Could you check a few things on this drawing? It's one solid part, dimensions in mm from its lowest x, y, z. A direction names the side the tool comes from. Coordinates: 2 decimals unless noted, no trailing zeros. Order: outer loops, then holes, each group sorted by start corner. A loop starts at its lowest first (then second) coordinate and runs counter-clockwise, first axis right, second up. Notation, with made-up numbers: (83, 6) - (101, 6) arc R21 ccw to (101, 30) - close; hole circle Ø2 at (-29, 72.5). An arc over 180 degrees is marked (long way). Return JSON: item names as keys, results as strings. Group by question number.
1) Imagine slicing it at A-A (y = 41.5). Write out the boundary of the cut face in (x, z).
2) Which directions (+Z, -Z, +X, -X, +Y, -Y) give clear straight access to the entire face, cutting with the end or side of a thin tool? Please do the marked faces 4 and 5.
3) If I drill on line 1 along X through (y, z) = (90, 13); line 2 along X through (y, z) = (18.5, 10.5); line 3 along Y through (x, z) = (27.5, 9.5), over which ranges is the centre line in solid material (lowest first)?
4) If we mould it in two halves opening along Y, with no side actions, what happens to the marked faces 1, 2 and 3? For each: pulls with the +Y half, pulls with the -Y half, needs draft (parallel to the pull), parting line crosses it, or undercut.
5) Imagine slicing it at B-B (x = 25.4). Write out the boundary of the cut face in (y, z), and give its area (3 significant figures).
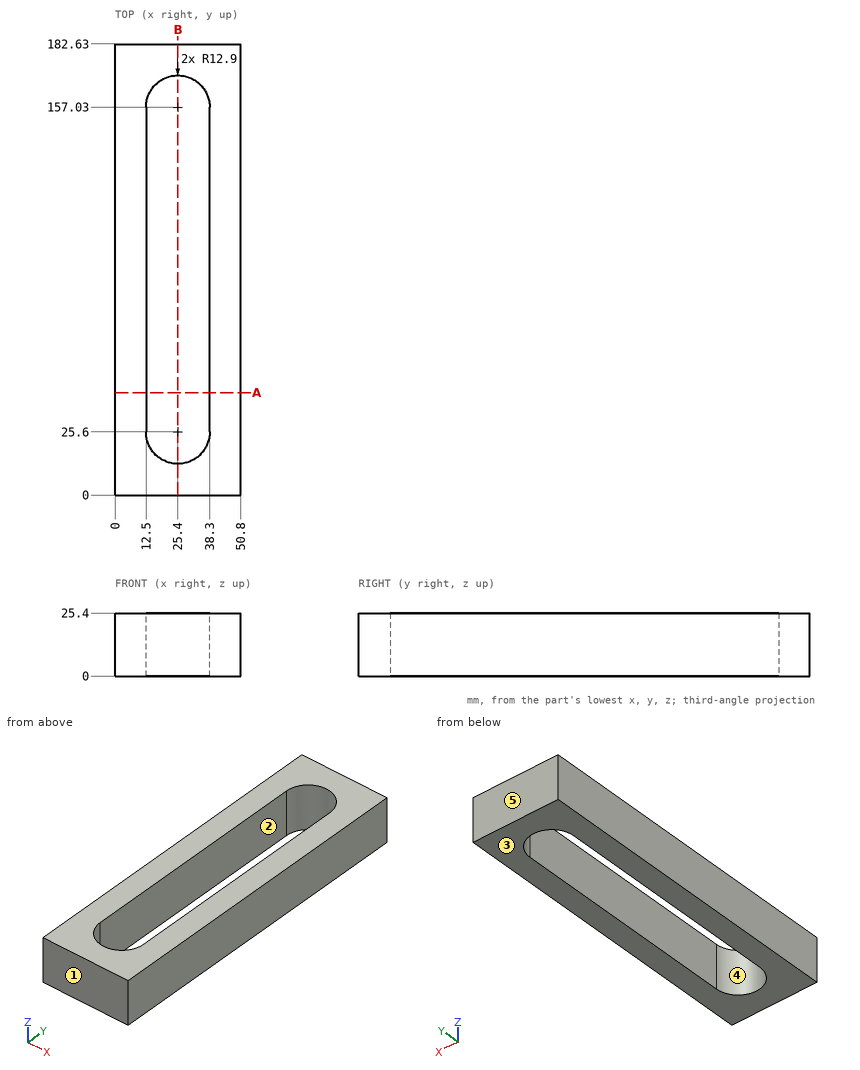
Calculated:
{
 "1": {"outline": "(0, 0) - (12.5, 0) - (12.5, 25.4) - (0, 25.4) - close; (38.3, 0) - (50.8, 0) - (50.8, 25.4) - (38.3, 25.4) - close"},
 "2": {"face 4": "+Z, -Z", "face 5": "+Z, -Z, +X, -X, +Y"},
 "3": {"line 1": "0 to 12.5, 38.3 to 50.8", "line 2": "0 to 14.63, 36.17 to 50.8", "line 3": "0 to 12.87, 169.76 to 182.63"},
 "4": {"face 1": "pulls with the -Y half", "face 2": "undercut", "face 3": "needs draft"},
 "5": {"outline": "(0, 0) - (12.7, 0) - (12.7, 25.4) - (0, 25.4) - close; (169.93, 0) - (182.63, 0) - (182.63, 25.4) - (169.93, 25.4) - close", "area": "645 mm2"}
}
